Design review of the part built by this model. Coordinates are the model's own, in mm. Face numbers are marked on the shaded views. A direction names the side the tool comes from. Coordinates: 2 decimals unless noted, no trailing zeros. Loops run counter-clockwise (first coordinate to the right, second up) from the corner with the lowest first, then second, coordinate; pieces in that order, holes last. Notation, with made-up numbers: (22.25, 21.25) -> (69.25, 21.25) arc R26 ccw to (69.25, 39.25) -> close; hole circle Ø11 at (24.5, 32). An arc over 180 degrees is marked (long way). One line per item, written item: value. Start each with the question number.
1. Add section D-D on z = -27. Write out the cut boundary in (x, y), plus the area to 3 significant figures.
2. Machinability: for the marked faces 1 and 2, which of the approach directions +Z, -Z, +X, -X, +Y, -Y give a long, thin tool a straight path to every point of the face, cutting with its end or side? Answer none if there is none.
3. Add section A-A on y = 8.25. Write out the cut boundary in (x, z).
4. Insertion check: pin 1 (1.5 mm diameter, centred on x = 16, y = 1.5, fed in from +Z); pin 2 (3 mm diameter, centred on x = 31.5, y = 5, fed in from +Z); pin 3 (3 mm diameter, centred on y = 7.5, z = -113, fed in from -X); pin 4 (4.5 mm diameter, centred on x = 6.5, z = -27, fed in from -Y). Each pin has a flat end and moves straight along its axis. Give the tip position at first contact, or say it passes through.
5. Add section B-B on z = -52. Write out the cut boundary in (x, y).
6. Add section C-C on x = 35. Write out the cut boundary in (y, z).
7. For probe 1 along X at (y, z) = (1.2, -27); probe 2 along Z at (x, y) = (25, 1.75); probe 3 along Z at (x, y) = (15, 2.5), list the stretches that pass through material, from the lowest coordinate up.
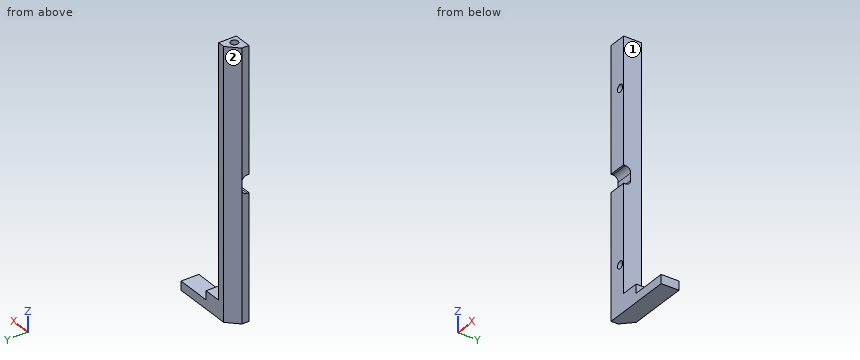
```python
from build123d import *

# Parameters (mm, degrees)
DODANIE_WYCI_GNI_CIE1_DEPTH = 10
SZKIC2_R                    = 2.1
WYTNIJ_WYCI_GNI_CIE1_DEPTH  = 4
SZKIC3_R                    = 2.1
WYTNIJ_WYCI_GNI_CIE2_DEPTH  = 4
SFAZOWANIE1_SIZE            = 6
SZKIC4_W                    = 10
SZKIC4_H                    = 10
WYTNIJ_WYCI_GNI_CIE3_DEPTH  = 4
ZAOKR_GLENIE1_R             = 3


with BuildPart() as part:
    # Szkic1 → Dodanie-wyciągnięcie1 (new body)
    with BuildSketch(Plane(origin=(0, 0, 0), x_dir=(1, 0, 0), z_dir=(0, 1, 0))):
        Polygon((0, 0), (0, 150), (40, 150), (40, 145), (20, 145), (20, 140), (10, 140), (10, 0), align=None)
    extrude(amount=DODANIE_WYCI_GNI_CIE1_DEPTH)

    # Szkic2 → Wytnij-wyciągnięcie1 (cut)
    with BuildSketch(Plane.XZ):
        with Locations(Location((7.2, -27, 0), (0, 0, 270))):
            Circle(SZKIC2_R)
        with Locations(Location((7.2, -123, 0), (0, 0, 270))):
            Circle(SZKIC2_R)
    extrude(amount=-WYTNIJ_WYCI_GNI_CIE1_DEPTH, mode=Mode.SUBTRACT)

    # Szkic3 → Wytnij-wyciągnięcie2 (cut)
    with BuildSketch(Plane.XY):
        with Locations((6, 4)):
            Circle(SZKIC3_R)
    extrude(amount=-WYTNIJ_WYCI_GNI_CIE2_DEPTH, mode=Mode.SUBTRACT)

    # Sfazowanie1
    sfazowanie1_edges = [part.edges().sort_by_distance(p)[0] for p in [
        (0, 10, -75),
    ]]
    chamfer(sfazowanie1_edges, length=SFAZOWANIE1_SIZE)

    # Szkic4 → Wytnij-wyciągnięcie3 (cut)
    with BuildSketch(Plane.XZ):
        with Locations((5, -75)):
            Rectangle(SZKIC4_W, SZKIC4_H)
    extrude(amount=-WYTNIJ_WYCI_GNI_CIE3_DEPTH, mode=Mode.SUBTRACT)

    # Zaokrąglenie1
    zaokr_glenie1_edges = [part.edges().sort_by_distance(p)[0] for p in [
        (5, 4, -70),
        (5, 4, -80),
    ]]
    fillet(zaokr_glenie1_edges, radius=ZAOKR_GLENIE1_R)


solid = part.part
```
Worked answers:
1. outline: (0, 0) -> (5.1, 0) -> (5.1, 4) -> (9.3, 4) -> (9.3, 0) -> (10, 0) -> (10, 10) -> (6, 10) -> (0, 4) -> close
1. area: 65.2 mm²
2. face 1: +Z, +X, +Y, -Y
2. face 2: +Z, -Z, -X, +Y
3. outline: (4.25, -150) -> (40, -150) -> (40, -145) -> (20, -145) -> (20, -140) -> (10, -140) -> (10, 0) -> (4.25, 0) -> close
4. pin 1: stops at z = -140
4. pin 2: stops at z = -145
4. pin 3: stops at x = 2
4. pin 4: stops at y = 0
5. outline: (0, 0) -> (10, 0) -> (10, 10) -> (6, 10) -> (0, 4) -> close
6. outline: (0, -150) -> (10, -150) -> (10, -145) -> (0, -145) -> close
7. probe 1: x = 0 to 5.1, 9.3 to 10
7. probe 2: z = -150 to -145
7. probe 3: z = -150 to -140
